Geometry: final body of the model. Coordinates: model frame, mm. A direction names the side the tool comes from. Give positions to 0.01 mm unless a question says otherwise; leave off trailing zeros. Write each loop counter-clockwise with the first axis right and the second up, starting at its lowest first coordinate (ties: lowest second). Pieces come first, ordered by that corner, then holes.
```python
from build123d import *

# Parameters (mm, degrees)
SKETCH1_W           = 50
SKETCH1_H           = 30
BOSS_EXTRUDE1_DEPTH = 16
SKETCH2_W           = 40.5
SKETCH2_H           = 20.5
CUT_EXTRUDE1_DEPTH  = 61.464865831
SKETCH3_W           = 5.361453717
SKETCH3_H           = 2.1
SKETCH3_W_2         = 6
CUT_EXTRUDE2_DEPTH  = 1.25
SKETCH5_W           = 30
SKETCH5_H           = 5.881320982
BOSS_EXTRUDE2_DEPTH = 4
SKETCH4_R           = 2.25
CUT_EXTRUDE3_DEPTH  = 64.812224534
CUT_EXTRUDE4_DEPTH  = 64.812224534
FILLET1_R           = 1
FILLET2_R           = 2
FILLET3_R           = 2


with BuildPart() as part:
    # Sketch1 → Boss-Extrude1 (new body)
    with BuildSketch(Plane(origin=(0, 0, 0), x_dir=(1, 0, 0), z_dir=(0, 1, 0))):
        with Locations((25, 15)):
            Rectangle(SKETCH1_W, SKETCH1_H)
    extrude(amount=BOSS_EXTRUDE1_DEPTH)

    # Sketch2 → Cut-Extrude1 (cut, through all)
    with BuildSketch(Plane(origin=(0, 16, 0), x_dir=(1, 0, 0), z_dir=(0, 1, 0))):
        with Locations((25, 15)):
            Rectangle(SKETCH2_W, SKETCH2_H)
    extrude(amount=-CUT_EXTRUDE1_DEPTH, mode=Mode.SUBTRACT)

    # Sketch3 → Cut-Extrude2 (cut)
    with BuildSketch(Plane.XZ):
        with Locations((2.069273142, -15)):
            Rectangle(SKETCH3_W, SKETCH3_H)
        with Locations((47.362234217, -15)):
            Rectangle(SKETCH3_W_2, SKETCH3_H)
    extrude(amount=-CUT_EXTRUDE2_DEPTH, mode=Mode.SUBTRACT)

    # Sketch5 → Boss-Extrude2 (add)
    with BuildSketch(Plane(origin=(50, 0, 0), x_dir=(0, 0, -1), z_dir=(1, 0, 0))):
        with Locations((15, 4.219150797)):
            Rectangle(SKETCH5_W, SKETCH5_H)
    boss_extrude2 = extrude(amount=BOSS_EXTRUDE2_DEPTH)

    # Mirror1: Boss-Extrude2 across plane
    add(boss_extrude2.mirror(Plane(origin=(25, 0, 0), x_dir=(0, 0, 1), z_dir=(1, 0, 0))))

    # Sketch4 → Cut-Extrude3 (cut, through all)
    with BuildSketch(Plane.XZ):
        with Locations(Location((50.65, -20.55, 0), (0, 0, 253.208552885))):
            Circle(SKETCH4_R)
        with Locations(Location((-0.65, -20.55, 0), (0, 0, 286.791447115))):
            Circle(SKETCH4_R)
        with Locations(Location((50.65, -9.45, 0), (0, 0, 253.208552885))):
            Circle(SKETCH4_R)
        with Locations(Location((-0.65, -9.45, 0), (0, 0, 286.791447115))):
            Circle(SKETCH4_R)
    extrude(amount=-CUT_EXTRUDE3_DEPTH, mode=Mode.SUBTRACT)

    # Sketch7 → Cut-Extrude4 (cut, through all)
    with BuildSketch(Plane(origin=(50, 0, 0), x_dir=(0, 0, -1), z_dir=(1, 0, 0))):
        Polygon((26.03322218, 11), (20, 11), (20, 19.253471802), (25.386984847, 19.253471802), (25.386984847, 14.530939497), (28.241616166, 14.530939497), (28.241616166, 11), (28.241616166, 8.880902809), (26.03322218, 8.880902809), align=None)
    cut_extrude4 = extrude(amount=-CUT_EXTRUDE4_DEPTH, mode=Mode.SUBTRACT)

    # Mirror2: Cut-Extrude4 across plane
    add(cut_extrude4.mirror(Plane(origin=(0, 0, -15), x_dir=(1, 0, 0), z_dir=(0, 0, -1))), mode=Mode.SUBTRACT)

    # Fillet1
    fillet1_edges = [part.edges().sort_by_distance(p)[0] for p in [
        (25, 0, -30),
        (25, 0, 0),
        (25, 0, -4.75),
        (25, 0, -25.25),
        (25, 16, 0),
        (25, 16, -30),
    ]]
    fillet(fillet1_edges, radius=FILLET1_R)

    # Fillet2
    fillet2_edges = [part.edges().sort_by_distance(p)[0] for p in [
        (-4, 4.219150797, -30),
        (-4, 4.219150797, 0),
        (54, 4.219150797, 0),
        (54, 4.219150797, -30),
    ]]
    fillet(fillet2_edges, radius=FILLET2_R)

    # Fillet3
    fillet3_edges = [part.edges().sort_by_distance(p)[0] for p in [
        (1.531742423, 13.5, -10),
        (4.75, 13.5, -10),
        (1.531742423, 13.5, -20),
        (4.75, 13.5, -20),
        (45.25, 13.5, -10),
        (48.468257577, 13.5, -10),
        (45.25, 13.5, -20),
        (48.468257577, 13.5, -20),
    ]]
    fillet(fillet3_edges, radius=FILLET3_R - 0.0001)  # a hair under: the kernel refuses the full size


solid = part.part
```
Item 1: Reachability of faces 4 (the face through (-2, 7.16, -15)), 5 (the face through (50, 1, -13)), 6 (the face through (25, 8.881, -27)), 7 (the face through (48, 1, -16.05)), 8 (the face through (1.84, 13.46, -10.22)) from +Z, -Z, +X, -X, +Y, -Y: full face, straight path, thin tool, end or side. Return the list, or none.
Found:
face 4: +Z, -Z, -X, +Y
face 5: +Z, -Z, +X, -Y
face 6: +X, -X
face 7: +X, -X, -Y
face 8: -X, +Y
Item 2: Line query: L1, parallel to X at y = 6, z = -9.45; L2, parallel to Z at x = -0.65, y = 3.5; L3, parallel to Z at x = 11, y = 9. Output: solid intervals per line, ascending.
Found:
L1: x = -4 to -2.9, 1.6 to 4.75, 45.25 to 48.4, 52.9 to 54
L2: z = -30 to -22.8, -18.3 to -11.7, -7.2 to 0
L3: z = -30 to -28.24, -26.03 to -25.25, -4.75 to -3.97, -1.76 to 0
Item 3: Pin query (flat end, axial travel): pin 1 Ø0.7 at (x, y) = (34.5, 15.5) entering from -Z; pin 2 Ø1.5 at (y, z) = (10.5, -15) entering from +X; pin 3 Ø4.5 at (x, z) = (-2.5, -14) entering from +Y. Return the tip coordinate at first contact, or that it passes through.
Found:
pin 1: stops at z = -29.99
pin 2: stops at x = 50
pin 3: stops at y = 7.16
Item 4: Section B-B, the plane z = -20.55. Return the cut outline in (x, y), plus the area to 3 significant figures.
Found:
outline: (-4, 1.28) - (-2.9, 1.28) - (-2.9, 7.16) - (-4, 7.16) - close; (1.6, 0) - (4.75, 0) - (4.75, 11) - (1.6, 11) - close; (45.25, 0) - (48.4, 0) - (48.4, 11) - (45.25, 11) - close; (52.9, 1.28) - (54, 1.28) - (54, 7.16) - (52.9, 7.16) - close
area: 82.2 mm2
Item 5: Section A-A, the plane x = 21. Return the cut outline in (y, z).
Found:
outline: (0, -29) arc R1 ccw to (1, -30) - (15, -30) arc R1 ccw to (16, -29) - (16, -25.39) - (14.53, -25.39) - (14.53, -28.24) - (8.88, -28.24) - (8.88, -26.03) - (11, -26.03) - (11, -25.25) - (1, -25.25) arc R1 ccw to (0, -26.25) - close; (0, -3.75) arc R1 ccw to (1, -4.75) - (11, -4.75) - (11, -3.97) - (8.88, -3.97) - (8.88, -1.76) - (14.53, -1.76) - (14.53, -4.61) - (16, -4.61) - (16, -1) arc R1 ccw to (15, 0) - (1, 0) arc R1 ccw to (0, -1) - close
Item 6: Pull-direction query (Z, two-part tool) for faces 1 (the face through (53.4, 4.26, -0.57)), 2 (the face through (48.16, 13.46, -10.22)), 3 (the face through (2, 16, -15)); classes: +Z half, -Z half, draft (parallel to the pull), parting line (faces both ways), or undercut.
Found:
face 1: +Z half
face 2: undercut
face 3: draft
Item 7: Section D-D, the plane z = -13. Return the cut outline in (x, y), plus the area to 3 significant figures.
Found:
outline: (-4, 1.28) - (0, 1.28) - (0, 0) - (4.75, 0) - (4.75, 16) - (0, 16) - (0, 7.16) - (-4, 7.16) - close; (45.25, 0) - (50, 0) - (50, 1.28) - (54, 1.28) - (54, 7.16) - (50, 7.16) - (50, 16) - (45.25, 16) - close
area: 199 mm2
Item 8: Section C-C, the plane x = 50.65. Return the cut outline in (y, z).
Found:
outline: (1.28, -30) - (7.16, -30) - (7.16, -22.8) - (1.28, -22.8) - close; (1.28, -18.3) - (7.16, -18.3) - (7.16, -11.7) - (1.28, -11.7) - close; (1.28, -7.2) - (7.16, -7.2) - (7.16, 0) - (1.28, 0) - close
